from build123d import *

# Parameters (mm, degrees)
RESSALTO_EXTRUS_O1_DEPTH = 20
ESBO_O2_R                = 2.75
CORTE_EXTRUS_O1_DEPTH    = 2


with BuildPart() as part:
    # Esboço1 → Ressalto-extrusão1 (new body)
    with BuildSketch(Plane(origin=(0, 0, 0), x_dir=(1, 0, 0), z_dir=(0, 1, 0))):
        with BuildLine():
            Line((-0.521579636, 13.959411341), (-2.612148901, -5.931026567))
            Line((-2.612148901, -5.931026567), (-4.601192692, -5.72196964))
            Line((-4.601192692, -5.72196964), (-2.510623427, 14.168468267))
            ThreePointArc((-2.510623427, 14.168468267), (62.394563373, 69.6027347), (121.149734086, 7.687703545))
            Line((121.149734086, 7.687703545), (121.149734086, -32.312296455))
            Line((121.149734086, -32.312296455), (119.149734086, -32.312296455))
            Line((119.149734086, -32.312296455), (119.149734086, 7.687703545))
            ThreePointArc((119.149734086, 7.687703545), (62.289891461, 67.60547563), (-0.521579636, 13.959411341))
        make_face()
    extrude(amount=RESSALTO_EXTRUS_O1_DEPTH)

    # Esboço2 → Corte-extrusão1 (cut)
    with BuildSketch(Plane(origin=(121.149734086, 0, 0), x_dir=(0, 0, -1), z_dir=(1, 0, 0))):
        with Locations((-24.812296455, 10)):
            Circle(ESBO_O2_R)
    extrude(amount=-CORTE_EXTRUS_O1_DEPTH, mode=Mode.SUBTRACT)


solid = part.part
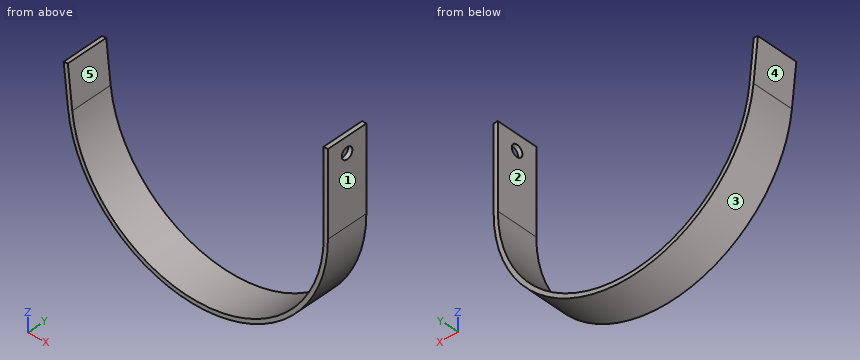
Can you work these out from the model? Positions are in its coordinate system, mm. Face numbers are marked on the shaded views. A direction names the side the tool comes from. Give positions to 0.01 mm unless a question says otherwise; leave off trailing zeros. Write each loop counter-clockwise with the first axis right and the second up, starting at its lowest first coordinate (ties: lowest second). Pieces come first, ordered by that corner, then holes. Notation, with made-up numbers: (-12.75, -1) -> (29.25, -1) arc R22 ccw to (29.25, 35) -> close; hole circle Ø4 at (85, 0). An arc over 180 degrees is marked (long way). Answer as a JSON object with one key per item and string values. Group by question number.
Item 1: Suppose I cut it at B-B (z = -52.5). Please give me the cut outline in (x, y).
Item 2: We'd pull the mould along X, two halves only. Please class the marked faces 3, 4 and 5: +X half, -X half, draft (parallel to the pull), parting line (faces both ways), or undercut.
Item 3: For the marked faces 1 and 2, which set-ups out of +Z, -Z, +X, -X, +Y, -Y let a thin tool reach every point of the face, with its end or its side?
Item 4: Please list where these lines run through material, in increasing order: line 1 (X direction, y = 8, z = 17); line 2 (X direction, y = 7.75, z = -50); line 3 (X direction, y = 5.25, z = -62.5). Write a range as [from, to].
Item 5: Suppose I cut it at D-D (x = 30). Please give me the cut outline in (y, z).
Item 6: Suppose I cut it at C-C (z = -3). Please give me the cut outline in (x, y), plus the area to 3 significant figures.
Item 7: I'm going to push flat-ended pins straight in: P1, Ø12, axis at x = 41, z = -54.5, coming from the +Y side; P2, Ø10, axis at x = 14.5, y = 10.5, coming from the -Z side; P3, Ø10, axis at y = 8, z = 13, coming from the -X side; P4, Ø3, axis at x = 15, y = 10, coming from the +Z side. Where does each tip first touch, or does it pass through?
Item 8: Suppose I cut it at A-A (y = 10). Please give me the cut outline in (x, z), plus the area to 3 significant figures.
Findings:
{
 "1": {"outline": "(16.3, 0) -> (19.25, 0) -> (19.25, 20) -> (16.3, 20) -> close; (99.05, 0) -> (102, 0) -> (102, 20) -> (99.05, 20) -> close"},
 "2": {"face 3": "parting line", "face 4": "-X half", "face 5": "undercut"},
 "3": {"face 1": "+Z, -Z, +X, +Y, -Y", "face 2": "+Z, +Y, -Y"},
 "4": {"line 1": "x = [119.15, 121.15]", "line 2": "x = [13.83, 16.61], [101.69, 104.47]", "line 3": "x = [30.17, 34.74], [83.55, 88.13]"},
 "5": {"outline": "(0, -62.41) -> (20, -62.41) -> (20, -60.13) -> (0, -60.13) -> close"},
 "6": {"outline": "(-3.68, 0) -> (-1.67, 0) -> (-1.67, 20) -> (-3.68, 20) -> close; (119.15, 0) -> (121.15, 0) -> (121.15, 20) -> (119.15, 20) -> close", "area": "80.2 mm²"},
 "7": {"P1": "passes through", "P2": "stops at z = -55.35", "P3": "stops at x = 119.15", "P4": "stops at z = -46.62"},
 "8": {"outline": "(-4.6, 5.72) -> (-2.51, -14.17) arc R62 ccw to (121.15, -7.69) -> (121.15, 22.06) -> (119.15, 22.06) -> (119.15, -7.69) arc R60 cw to (-0.52, -13.96) -> (-2.61, 5.93) -> close; (119.15, 27.56) -> (121.15, 27.56) -> (121.15, 32.31) -> (119.15, 32.31) -> close", "area": "479 mm²"}
}
